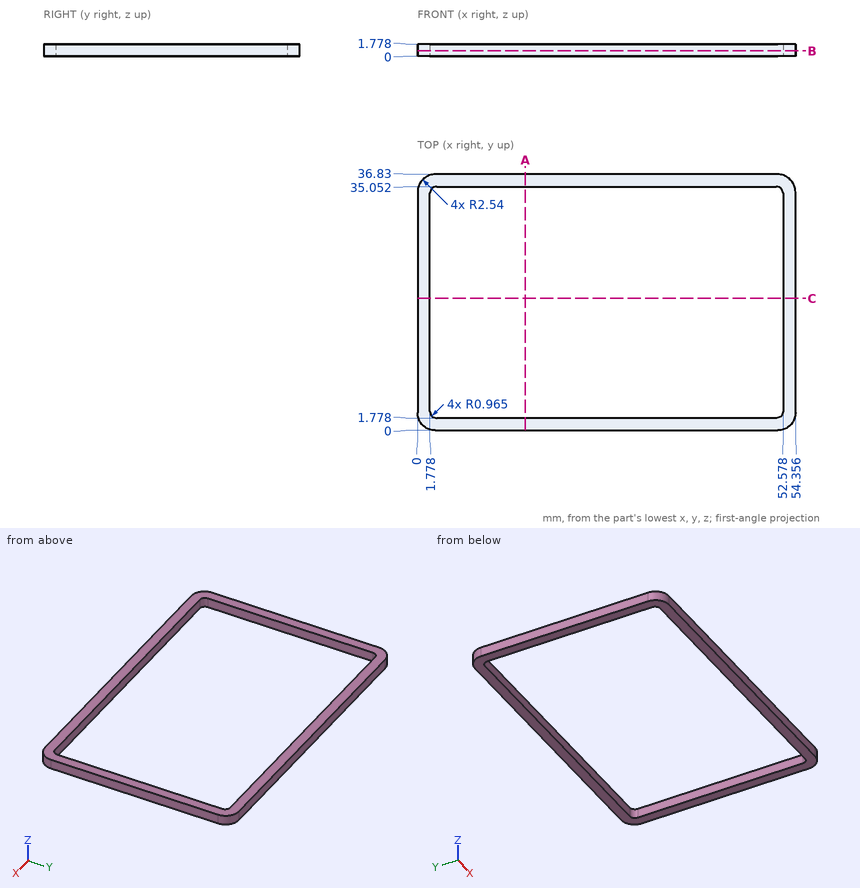
Answer from the drawing. Dimensions are ordinates in mm from the lowest x, y and z of the part. Coordinates: 2 decimals unless noted, no trailing zeros. Write each loop counter-clockwise with the first axis right and the second up, starting at its lowest first coordinate (ties: lowest second). Pieces come first, ordered by that corner, then holes. Notation, with made-up numbers: M -4,30.25 L 40,30.25 A13 ccw 40,51.25 Z; hole C 67.5,10 d10. An arc over 180 degrees is marked long. Use one line per item in the form item = value. Start each with the question number.
1. The part is cut by section A-A (x = 15.5). Give the vertices of the cut face in (y, z).
2. Straight lines are drawn through the part: probe 1 along X at (y, z) = (24.5, 0.65); probe 2 along Y at (x, z) = (33, 0.2). For each, find the intervals that lie inside material, in ascending order. Write a range as from..to.
3. The part is cut by section C-C (y = 19). Give the vertices of the cut face in (x, z).
4. This flat-tipped pin is pushed along its axis until it touches: P1, Ø8, axis at x = 7, y = 25, coming from the +Z side. Where does it stop, or does it pass through?
5. The part is cut by section B-B (z = 0.8). Give the vertices of the cut face in (x, y) (1 decimal), plus the area to 3 significant figures.
Evaluation:
q1.outline = M 0,0 L 1.78,0 L 1.78,1.78 L 0,1.78 Z; M 35.05,0 L 36.83,0 L 36.83,1.78 L 35.05,1.78 Z
q2.probe_1 = 0..1.78, 52.58..54.36
q2.probe_2 = 0..1.78, 35.05..36.83
q3.outline = M 0,0 L 1.78,0 L 1.78,1.78 L 0,1.78 Z; M 52.58,0 L 54.36,0 L 54.36,1.78 L 52.58,1.78 Z
q4.P1 = through
q5.outline = M 0,2.5 A2.5 ccw 2.5,0 L 51.8,0 A2.5 ccw 54.4,2.5 L 54.4,34.3 A2.5 ccw 51.8,36.8 L 2.5,36.8 A2.5 ccw 0,34.3 Z; hole M 1.8,2.7 A1 ccw 2.7,1.8 L 51.6,1.8 A1 ccw 52.6,2.7 L 52.6,34.1 A1 ccw 51.6,35.1 L 2.7,35.1 A1 ccw 1.8,34.1 Z
q5.area = 307 mm^2
